The model under review builds one solid part; all positions refer to its coordinate system, in mm. A direction names the side the tool comes from. Round coordinates to 2 decimals unless told otherwise and drop trailing zeros. Loops run counter-clockwise (first coordinate to the right, second up) from the corner with the lowest first, then second, coordinate; pieces in that order, holes last. Notation, with made-up numbers: (75.5, 76.25) -> (79.5, 76.25) arc R28 ccw to (79.5, 107.25) -> close; hole circle Ø3 at (26.5, -32). An arc over 180 degrees is marked (long way). Write each question's results on one line, items separated by ' | '. Start each with the question number.
Item 1: Tool access review of faces 1 (the cylindrical face through (11.923, 3.755, 242.27)), 2 (the flat face through (0, 0, -410)), 3 (the flat face through (-11.5, 5.9, -50)): name each direction out of +Z, -Z, +X, -X, +Y, -Y from which nothing blocks a thin tool from reaching the whole face with its end or side.
Item 2: We need section A-A (x = 0). Give the boundary of the cut face in (y, z).
Item 3: Clearance check with flat-ended pins moving along their axes: pin 1 Ø5 at (y, z) = (-6, 3.5) entering from +X; pin 2 Ø4 at (x, y) = (-19.5, -3.5) entering from +Z; pin 3 Ø1 at (y, z) = (-14, 227) entering from +X; pin 4 Ø8 at (y, z) = (14.5, 210.5) entering from +X. State where each tip first meets the part, or that it passes through.
Item 4: We need section C-C (z = -285.5). Give the boundary of the cut face in (x, y).
Item 5: For L1, parallel to Z at x = -15.5, y = 9.5; L2, parallel to X at y = 1.5, z = -272.5; L3, parallel to X at y = -1, z = 234, list the stretches that pass through material, from the lowest coordinate up. Write a range as from..to.
from build123d import *

# Parameters (mm, degrees)
SKETCH1_R                = 25
SKETCH1_R_2              = 12.5
BOSS_EXTRUDE1_DEPTH      = 50
BOSS_EXTRUDE1_DEPTH_BACK = 50
SKETCH3_R                = 12.5
BOSS_EXTRUDE3_DEPTH      = 390
BOSS_EXTRUDE3_DEPTH_BACK = 460


with BuildPart() as part:
    # Sketch1 → Boss-Extrude1 (new body, two sides)
    with BuildSketch(Plane.XY) as boss_extrude1_sk:
        Circle(SKETCH1_R)
        Circle(SKETCH1_R_2, mode=Mode.SUBTRACT)
    extrude(amount=BOSS_EXTRUDE1_DEPTH)
    extrude(boss_extrude1_sk.sketch, amount=-BOSS_EXTRUDE1_DEPTH_BACK)

    # Sketch3 → Boss-Extrude3 (add, two sides)
    with BuildSketch(Plane.XY.offset(50)) as boss_extrude3_sk:
        Circle(SKETCH3_R)
    extrude(amount=BOSS_EXTRUDE3_DEPTH)
    extrude(boss_extrude3_sk.sketch, amount=-BOSS_EXTRUDE3_DEPTH_BACK)


solid = part.part
Here are the results:
1) face 1: +Z | face 2: -Z, +X, -X, +Y, -Y | face 3: -Z
2) outline: (-25, -50) -> (-12.5, -50) -> (-12.5, -410) -> (12.5, -410) -> (12.5, -50) -> (25, -50) -> (25, 50) -> (12.5, 50) -> (12.5, 440) -> (-12.5, 440) -> (-12.5, 50) -> (-25, 50) -> close
3) pin 1: stops at x = 24.75 | pin 2: stops at z = 50 | pin 3: passes through | pin 4: stops at x = 6.78
4) outline: circle Ø25 at (0, 0)
5) L1: z = -50..50 | L2: x = -12.41..12.41 | L3: x = -12.46..12.46
